```python
from build123d import *

# Parameters (mm, degrees)
SKETCH1_R               = 3.2
SKETCH1_W               = 26.7
SKETCH1_H               = 32.3
BOSS_EXTRUDE2_DEPTH     = 10
CUT_EXTRUDE1_DEPTH      = 68.219866013
SKETCH3_W               = 36.125771517
SKETCH3_H               = 4
CUT_EXTRUDE2_DEPTH      = 77.38869507
CUT_EXTRUDE3_REACH      = 60.207
CUT_EXTRUDE3_END_RADIUS = 3.2
SKETCH4_W               = 4.857578305
SKETCH4_H               = 4
CUT_EXTRUDE4_REACH      = 60.207
CUT_EXTRUDE4_END_RADIUS = 3.2
SKETCH5_W               = 4.857578305
SKETCH5_H               = 4
CUT_EXTRUDE5_REACH      = 60.207
CUT_EXTRUDE5_END_RADIUS = 3.2
SKETCH6_W               = 4.857578305
SKETCH6_H               = 4
CUT_EXTRUDE6_REACH      = 60.207
CUT_EXTRUDE6_END_RADIUS = 3.2
SKETCH7_W               = 4.857578305
SKETCH7_H               = 4
SKETCH8_W               = 10.205315409
SKETCH8_H               = 1.2
SKETCH8_W_2             = 1.2
SKETCH8_H_2             = 16.7681893
BOSS_EXTRUDE3_DEPTH     = 4
CUT_EXTRUDE7_DEPTH      = 52.578594453
SKETCH10_W              = 10.205315409
SKETCH10_H              = 0.6
BOSS_EXTRUDE4_DEPTH     = 1.2
CHAMFER1_SIZE           = 1.2
SKETCH12_W              = 10.205315409
SKETCH12_H              = 0.6
BOSS_EXTRUDE5_DEPTH     = 1.2
CHAMFER2_SIZE           = 1.2
CUT_EXTRUDE8_DEPTH      = 53.070638614
CUT_EXTRUDE8_DEPTH_BACK = 3


with BuildPart() as part:
    # Sketch1 → Boss-Extrude2 (new body)
    with BuildSketch(Plane(origin=(0, 0, 0), x_dir=(1, 0, 0), z_dir=(0, 1, 0))):
        with BuildLine():
            Line((-34.405486348, 30.435899661), (-24.03957695, 12.074655042))
            Line((-24.03957695, 12.074655042), (-24.03957695, -0.625344958))
            Line((-24.03957695, -0.625344958), (-34.405486348, -18.986589577))
            ThreePointArc((-34.405486348, -18.986589577), (-33.407763681, -24.841890549), (-27.552462708, -23.844167882))
            Line((-27.552462708, -23.844167882), (-13.03957695, -11.625344958))
            Line((-13.03957695, -11.625344958), (-5.93957695, -11.625344958))
            Line((-5.93957695, -11.625344958), (8.573308809, -23.844167882))
            ThreePointArc((8.573308809, -23.844167882), (14.428609781, -24.841890549), (15.426332449, -18.986589577))
            Line((15.426332449, -18.986589577), (5.06042305, -0.625344958))
            Line((5.06042305, -0.625344958), (5.06042305, 12.074655042))
            Line((5.06042305, 12.074655042), (15.426332449, 30.435899661))
            ThreePointArc((15.426332449, 30.435899661), (14.428609781, 36.291200634), (8.573308809, 35.293477966))
            Line((8.573308809, 35.293477966), (-5.93957695, 23.074655042))
            Line((-5.93957695, 23.074655042), (-13.03957695, 23.074655042))
            Line((-13.03957695, 23.074655042), (-27.552462708, 35.293477966))
            ThreePointArc((-27.552462708, 35.293477966), (-33.407763681, 36.291200634), (-34.405486348, 30.435899661))
        make_face()
        with Locations(Location((-30.978974528, 32.864688814, 0), (0, 0, 270))):
            Circle(SKETCH1_R, mode=Mode.SUBTRACT)
        with Locations(Location((11.999820629, 32.864688814, 0), (0, 0, 90))):
            Circle(SKETCH1_R, mode=Mode.SUBTRACT)
        with Locations(Location((-30.978974528, -21.415378729, 0), (0, 0, 90))):
            Circle(SKETCH1_R, mode=Mode.SUBTRACT)
        with Locations(Location((11.999820629, -21.415378729, 0), (0, 0, 270))):
            Circle(SKETCH1_R, mode=Mode.SUBTRACT)
        with BuildLine():
            Line((-24.03957695, 23.074655042), (-14.592234654, 23.074655042))
            Line((-14.592234654, 23.074655042), (-26.808244007, 33.359670553))
            ThreePointArc((-26.808244007, 33.359670553), (-28.363078678, 29.578796408), (-32.396270044, 28.911048286))
            Line((-32.396270044, 28.911048286), (-24.03957695, 14.108749692))
            Line((-24.03957695, 14.108749692), (-24.03957695, 23.074655042))
        make_face(mode=Mode.SUBTRACT)
        with Locations((-9.48957695, 5.724655042)):
            Rectangle(SKETCH1_W, SKETCH1_H, mode=Mode.SUBTRACT)
        with BuildLine():
            Line((5.06042305, 23.074655042), (5.06042305, 14.108749692))
            Line((5.06042305, 14.108749692), (13.417116145, 28.911048286))
            ThreePointArc((13.417116145, 28.911048286), (9.383924779, 29.578796408), (7.829090108, 33.359670553))
            Line((7.829090108, 33.359670553), (-4.386919245, 23.074655042))
            Line((-4.386919245, 23.074655042), (5.06042305, 23.074655042))
        make_face(mode=Mode.SUBTRACT)
        with BuildLine():
            Line((-24.03957695, -11.625344958), (-14.592234654, -11.625344958))
            Line((-14.592234654, -11.625344958), (-26.808244007, -21.910360468))
            ThreePointArc((-26.808244007, -21.910360468), (-28.363078678, -18.129486324), (-32.396270044, -17.461738202))
            Line((-32.396270044, -17.461738202), (-24.03957695, -2.659439608))
            Line((-24.03957695, -2.659439608), (-24.03957695, -11.625344958))
        make_face(mode=Mode.SUBTRACT)
        with BuildLine():
            Line((7.829090108, -21.910360468), (-4.386919245, -11.625344958))
            Line((-4.386919245, -11.625344958), (5.06042305, -11.625344958))
            Line((5.06042305, -11.625344958), (5.06042305, -2.659439608))
            Line((5.06042305, -2.659439608), (13.417116145, -17.461738202))
            ThreePointArc((13.417116145, -17.461738202), (9.383924779, -18.129486324), (7.829090108, -21.910360468))
        make_face(mode=Mode.SUBTRACT)
    extrude(amount=BOSS_EXTRUDE2_DEPTH)

    # Sketch2 → Cut-Extrude1 (cut, through all)
    with BuildSketch(Plane(origin=(20, 0, 0), x_dir=(0, 0, -1), z_dir=(1, 0, 0))):
        Polygon((-18.986589577, 5), (-18.986589577, 7), (-0.625344958, 7), (-0.625344958, 5), (-0.625344958, 3), (-18.986589577, 3), align=None)
        Polygon((30.435899661, 7), (12.074655042, 7), (12.074655042, 5), (12.074655042, 3), (30.435899661, 3), (30.435899661, 5), align=None)
    extrude(amount=-CUT_EXTRUDE1_DEPTH, mode=Mode.SUBTRACT)

    # Sketch3 → Cut-Extrude2 (cut, through all)
    with BuildSketch(Plane.XY.offset(30)):
        with Locations((-9.489576949, 5)):
            Rectangle(SKETCH3_W, SKETCH3_H)
    extrude(amount=-CUT_EXTRUDE2_DEPTH, mode=Mode.SUBTRACT)

    # Cut-Extrude3: up to this cylinder (the profile starts outside it)
    cut_extrude3_end = Plane(origin=(-30.978974528, 5, 21.415378729), z_dir=(0, -1, 0)) * Cylinder(CUT_EXTRUDE3_END_RADIUS, 127.814, mode=Mode.PRIVATE)
    # Sketch4 → Cut-Extrude3 (cut, up to the surface)
    with BuildSketch(Plane(origin=(-27.552462708, 0, 0), x_dir=(0, 0, -1), z_dir=(1, 0, 0)), mode=Mode.PRIVATE) as cut_extrude3_sk1:
        with Locations((-21.415378729, 5)):
            Rectangle(SKETCH4_W, SKETCH4_H)
    cut_extrude3_tool1 = extrude(cut_extrude3_sk1.sketch, amount=-CUT_EXTRUDE3_REACH, mode=Mode.PRIVATE) - cut_extrude3_end
    add(cut_extrude3_tool1.solids().sort_by_distance((-27.552463, 5, 21.415379))[0], mode=Mode.SUBTRACT)

    # Cut-Extrude4: up to this cylinder (the profile starts outside it)
    cut_extrude4_end = Plane(origin=(11.999820629, 5, 21.415378729), z_dir=(0, -1, 0)) * Cylinder(CUT_EXTRUDE4_END_RADIUS, 127.814, mode=Mode.PRIVATE)
    # Sketch5 → Cut-Extrude4 (cut, up to the surface)
    with BuildSketch(Plane.ZY.offset(-8.573308809), mode=Mode.PRIVATE) as cut_extrude4_sk1:
        with Locations((21.415378729, 5)):
            Rectangle(SKETCH5_W, SKETCH5_H)
    cut_extrude4_tool1 = extrude(cut_extrude4_sk1.sketch, amount=-CUT_EXTRUDE4_REACH, mode=Mode.PRIVATE) - cut_extrude4_end
    add(cut_extrude4_tool1.solids().sort_by_distance((8.573309, 5, 21.415379))[0], mode=Mode.SUBTRACT)

    # Cut-Extrude5: up to this cylinder (the profile starts outside it)
    cut_extrude5_end = Plane(origin=(-30.978974528, 5, -32.864688814), z_dir=(0, -1, 0)) * Cylinder(CUT_EXTRUDE5_END_RADIUS, 127.814, mode=Mode.PRIVATE)
    # Sketch6 → Cut-Extrude5 (cut, up to the surface)
    with BuildSketch(Plane(origin=(-27.552462708, 0, 0), x_dir=(0, 0, -1), z_dir=(1, 0, 0)), mode=Mode.PRIVATE) as cut_extrude5_sk1:
        with Locations((32.864688814, 5)):
            Rectangle(SKETCH6_W, SKETCH6_H)
    cut_extrude5_tool1 = extrude(cut_extrude5_sk1.sketch, amount=-CUT_EXTRUDE5_REACH, mode=Mode.PRIVATE) - cut_extrude5_end
    add(cut_extrude5_tool1.solids().sort_by_distance((-27.552463, 5, -32.864689))[0], mode=Mode.SUBTRACT)

    # Cut-Extrude6: up to this cylinder (the profile starts outside it)
    cut_extrude6_end = Plane(origin=(11.999820629, 5, -32.864688814), z_dir=(0, -1, 0)) * Cylinder(CUT_EXTRUDE6_END_RADIUS, 127.814, mode=Mode.PRIVATE)
    # Sketch7 → Cut-Extrude6 (cut, up to the surface)
    with BuildSketch(Plane.ZY.offset(-8.573308809), mode=Mode.PRIVATE) as cut_extrude6_sk1:
        with Locations((-32.864688814, 5)):
            Rectangle(SKETCH7_W, SKETCH7_H)
    cut_extrude6_tool1 = extrude(cut_extrude6_sk1.sketch, amount=-CUT_EXTRUDE6_REACH, mode=Mode.PRIVATE) - cut_extrude6_end
    add(cut_extrude6_tool1.solids().sort_by_distance((8.573309, 5, -32.864689))[0], mode=Mode.SUBTRACT)

    # Sketch8 → Boss-Extrude3 (add)
    with BuildSketch(Plane(origin=(0, 3, 0), x_dir=(1, 0, 0), z_dir=(0, 1, 0))):
        with Locations((-9.489576949, 22.474655042)):
            Rectangle(SKETCH8_W, SKETCH8_H)
        with Locations((-9.489576949, -11.025344958)):
            Rectangle(SKETCH8_W, SKETCH8_H)
        with Locations((-23.43957695, 5.724655042)):
            Rectangle(SKETCH8_W_2, SKETCH8_H_2)
        with Locations((4.46042305, 5.724655042)):
            Rectangle(SKETCH8_W_2, SKETCH8_H_2)
    extrude(amount=BOSS_EXTRUDE3_DEPTH)

    # Sketch9 → Cut-Extrude7 (cut, through all)
    with BuildSketch(Plane(origin=(0, 3, 0), x_dir=(1, 0, 0), z_dir=(0, 1, 0))):
        Polygon((-27.717427746, 29.299754586), (-28.696368176, 28.605726031), (-30.707626394, 31.442643867), (-29.728685964, 32.136672421), align=None)
        Polygon((11.728472495, 31.442643867), (10.749532065, 32.136672421), (8.738273847, 29.299754586), (9.717214277, 28.605726031), align=None)
        Polygon((9.717214277, -16.898697434), (11.728472495, -19.735615269), (10.749532065, -20.429643824), (8.738273847, -17.592725989), align=None)
        Polygon((-30.707626394, -19.735615269), (-29.728685964, -20.429643824), (-27.717427746, -17.592725989), (-28.696368176, -16.898697434), align=None)
    extrude(amount=-CUT_EXTRUDE7_DEPTH, mode=Mode.SUBTRACT)

    # Sketch10 → Boss-Extrude4 (add)
    with BuildSketch(Plane.XY.offset(-21.874655042)):
        with Locations((-9.489576949, 6.7)):
            Rectangle(SKETCH10_W, SKETCH10_H)
    extrude(amount=BOSS_EXTRUDE4_DEPTH)

    # Chamfer1
    chamfer1_edges = [part.edges().sort_by_distance(p)[0] for p in [
        (-9.48957695, 6.4, -21.874655042),
    ]]
    chamfer(chamfer1_edges, length=CHAMFER1_SIZE - 0.0001)  # a hair under: the kernel refuses the full size

    # Sketch12 → Boss-Extrude5 (add)
    with BuildSketch(Plane(origin=(0, 0, 10.425344958), x_dir=(-1, 0, 0), z_dir=(0, 0, -1))):
        with Locations((9.489576949, 6.7)):
            Rectangle(SKETCH12_W, SKETCH12_H)
    extrude(amount=BOSS_EXTRUDE5_DEPTH)

    # Chamfer2
    chamfer2_edges = [part.edges().sort_by_distance(p)[0] for p in [
        (-9.48957695, 6.4, 10.425344958),
    ]]
    chamfer(chamfer2_edges, length=CHAMFER2_SIZE - 0.0001)  # a hair under: the kernel refuses the full size

    # Sketch13 → Cut-Extrude8 (cut, two sides: drawn at the far end of the back side and taken through both)
    with BuildSketch(Plane(origin=(0, 10, 0), x_dir=(1, 0, 0), z_dir=(0, 1, 0)).offset(-CUT_EXTRUDE8_DEPTH_BACK)):
        Polygon((-14.592234654, 23.074655042), (-13.392234654, 21.874655042), (-15.393970224, 21.874655042), (-16.593970224, 23.074655042), align=None)
        Polygon((-3.585183676, 21.874655042), (-2.385183676, 23.074655042), (-4.386919245, 23.074655042), (-5.586919245, 21.874655042), align=None)
        Polygon((-5.586919245, -10.425344958), (-3.585183676, -10.425344958), (-2.385183676, -11.625344958), (-4.386919245, -11.625344958), align=None)
        Polygon((-15.393970224, -10.425344958), (-16.593970224, -11.625344958), (-14.592234654, -11.625344958), (-13.392234654, -10.425344958), align=None)
    extrude(amount=CUT_EXTRUDE8_DEPTH + CUT_EXTRUDE8_DEPTH_BACK, mode=Mode.SUBTRACT)


solid = part.part
```
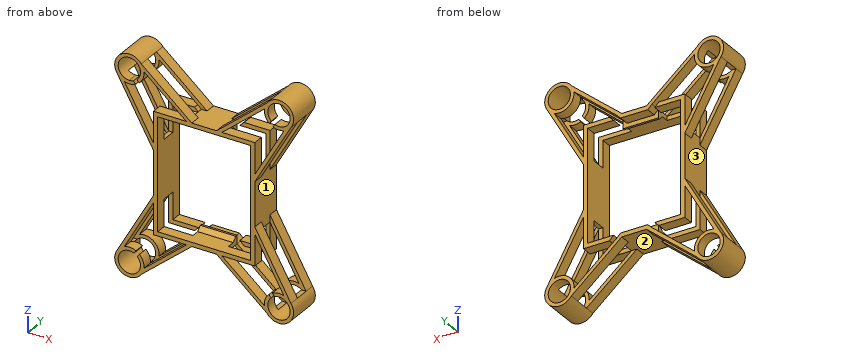
Could you check a few things on this model? Use its own coordinates, in mm. Face numbers are marked on the shaded views. Coordinates: 2 decimals unless noted, no trailing zeros. Loops run counter-clockwise (first coordinate to the right, second up) from the corner with the lowest first, then second, coordinate; pieces in that order, holes last. Notation, with made-up numbers: M -11,39.25 L 32,39.25 A19 cw 32,67.25 Z; hole C -26,-9 d4. An arc over 180 degrees is marked long. Put each result on its own line as item: value. Start each with the question number.
(1) Suppose I cut it at A-A on z = -9.5. Please give me the cut outline in (x, y), then the cut area to 3 significant figures.
(2) Will these pins go through, and if not, where does the flat tip stop? P1, Ø6, axis at x = -5, z = 4.5, coming from the -Y side; P2, Ø2.5, axis at y = 1, z = 9, coming from the +X side; P3, Ø6, axis at y = 6.5, z = -17, coming from the +X side; P4, Ø2.5, axis at x = -9.5, y = 8, coming from the +Z side.
(3) Suppose I cut it at C-C on x = -20. Count the separate pieces of the cut face and the enclosed holes in it, then the cut area to 3 significant figures.
(4) Thinking about a two-plate mould opening in X: for the marked faces 1, 2 and 3, which applies, pulls with the +X half, pulls with the -X half, needs draft (parallel to the pull), parting line crosses it, or undercut?
(5) I need wall thicknesses on line 1 (Y direction, x = -20, z = 11); line 2 (Z direction, x = -25.5, y = 8.25); line 3 (Z direction, x = -22, y = 9.25). Which ranges of each line are inside material? Lowest first, please. Write a range as from..to.
Solutions:
1. outline: M -24.04,0 L -22.84,0 L -22.84,10 L -24.04,10 Z; M 3.86,0 L 5.06,0 L 5.06,10 L 3.86,10 Z
1. area: 24.0 mm2
2. P1: passes through
2. P2: stops at x = 10.49
2. P3: stops at x = 9.51
2. P4: stops at z = 11.63
3. separate pieces: 8
3. enclosed holes: 0
3. area: 30.1 mm2
4. face 1: pulls with the +X half
4. face 2: undercut
4. face 3: pulls with the -X half
5. line 1: y = 0..3, 7..10
5. line 2: z = -33.57..-32.26, -16.7..-14.66, 3.21..5.25, 20.81..22.12
5. line 3: z = -30.62..-29.31, -23.07..-21.87, 10.43..11.63, 17.86..19.17
